Input: part model. Units: mm. Frame: model coordinates. A direction names the side the tool comes from. Coordinates: 2 decimals unless noted, no trailing zeros. Loops run counter-clockwise (first coordinate to the right, second up) from the corner with the lowest first, then second, coordinate; pieces in that order, holes last.
```python
from build123d import *

# Parameters (mm, degrees)
F1_DEPTH = 50
F3_R     = 1.8504510886
F4_DEPTH = 2.5
F5_R     = 3
F6_SIZE  = 1


with BuildPart() as f1:
    # F0 (on Front) → F1 (new body)
    with BuildSketch(Plane.XZ):
        Polygon((18.8134295464, 46.3255314994), (0, 0), (50, 0), (50, 5), (7.427160285, 5), (23.4459826963, 44.4441885448), align=None)
    extrude(amount=F1_DEPTH)

    # F3 (on offset) → F4 (join, symmetric)
    with BuildSketch(Plane.XZ.offset(25)):
        Polygon((28.7135801425, 5), (15.4365714906, 24.7220942724), (7.427160285, 5), align=None)
        with Locations((15.7413743436, 11.3711580634)):
            Circle(F3_R, mode=Mode.SUBTRACT)
    extrude(amount=F4_DEPTH, both=True)

    # F5
    f5_edges = [f1.edges().sort_by_distance(p)[0] for p in [
        (0, -25, 0),
        (18.07037, -27.5, 5),
        (11.431866, -27.5, 14.861047),
        (11.431866, -22.5, 14.861047),
        (18.07037, -22.5, 5),
        (7.42716, -38.75, 5),
        (7.42716, -11.25, 5),
    ]]
    fillet(f5_edges, radius=F5_R)

    # F6
    f6_edges = [f1.edges().sort_by_distance(p)[0] for p in [
        (18.81343, -25, 46.325531),
        (50, -25, 5),
    ]]
    chamfer(f6_edges, length=F6_SIZE)


solid = f1.part
```
Item 1: Contact query for flat-ended pins moving along their axis: P1, Ø4.5, axis at x = 15.74, z = 11.37, coming from the -Y side; P2, Ø12, axis at y = -30, z = 41, coming from the +X side; P3, Ø6, axis at x = 42.5, y = -6.5, coming from the +Z side. Output: stop coordinate, or through.
Result:
P1: stops at y = -27.5
P2: stops at x = 23.45
P3: stops at z = 5
Item 2: Mould query, pull axis Z, two halves, no side actions, for faces 1 (the face through (13.02, -21.6, 16.49)), 2 (the face through (11, -50, 15)), 3 (the face through (27, -25, 0)). Classes: +Z half, -Z half, draft (parallel to the pull), parting line (faces both ways), or undercut.
Result:
face 1: undercut
face 2: draft
face 3: -Z half
Item 3: Section query A-A (y = -15). Output: boundary loops of the cut face in (x, z), then the cut area to 3 significant figures.
Result:
outline: (1.68, 4.13) arc R3 ccw to (4.46, 0) - (50, 0) - (50, 4) - (49, 5) - (11.88, 5) arc R3 cw to (9.1, 9.13) - (23.45, 44.44) - (19.74, 45.95) - (18.44, 45.4) - close
area: 462 mm2
Item 4: Section query C-C (x = 45). Output: boundary loops of the cut face in (y, z).
Result:
outline: (-50, 0) - (0, 0) - (0, 5) - (-50, 5) - close
Item 5: Section query D-D (y = -24). Output: boundary loops of the cut face in (x, z).
Result:
outline: (1.68, 4.13) arc R3 ccw to (4.46, 0) - (50, 0) - (50, 4) - (49, 5) - (28.71, 5) - (15.44, 24.72) - (23.45, 44.44) - (19.74, 45.95) - (18.44, 45.4) - close; hole circle Ø3.7 at (15.74, 11.37)
Item 6: Line query: L1, parallel to Z at x = 34, y = -40.5; L2, parallel to Z at x = 23, y = -5.5; L3, parallel to X at y = -36.5, z = 20.5. Output: solid intervals per line, ascending.
Result:
L1: z = 0 to 5
L2: z = 0 to 5, 43.35 to 44.63
L3: x = 8.33 to 13.72
Item 7: Section query B-B (z = 6). Output: boundary loops of the cut face in (x, y), then the cut area to 3 significant figures.
Result:
outline: (2.44, -50) - (9.65, -50) - (9.65, -30.5) arc R2.24 cw to (11.88, -28.26) - (28.04, -28.26) - (28.04, -21.74) - (11.88, -21.74) arc R2.24 cw to (9.65, -19.5) - (9.65, 0) - (2.44, 0) - close
area: 483 mm2
Item 8: Reachability of faces 4 (the face through (13.02, -28.4, 16.49)), 5 (the face through (22.17, -25.08, 14.72)), 6 (the face through (20.42, -21.6, 5.86)) from +Z, -Z, +X, -X, +Y, -Y: full face, straight path, thin tool, end or side. Return the list, or none.
Result:
face 4: +X, -Y
face 5: +X, +Y, -Y
face 6: +X, +Y
